Can you work these out from the drawing? Everything is in mm from the part's minimum corner. Give positions to 0.01 mm unless a question says otherwise; leave off trailing zeros. Write each loop counter-clockwise with the first axis right and the second up, starting at its lowest first coordinate (ties: lowest second). Pieces come first, ordered by that corner, then holes. Notation, with made-up numbers: (9.5, 51) -> (15.5, 51) arc R26 cw to (15.5, 79) -> close; hole circle Ø5 at (15.5, 79). An arc over 180 degrees is marked (long way). Return JSON: item names as keys, results as strings.
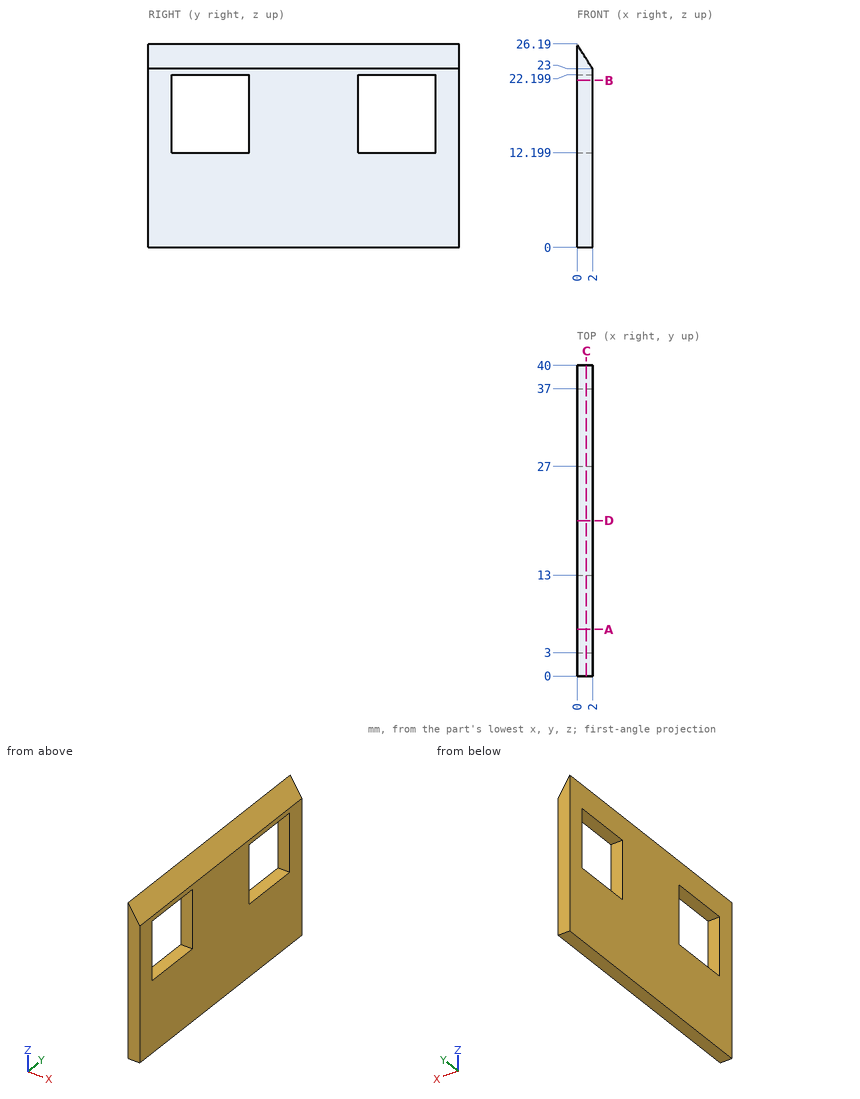
1. If I drill on line 1 (Y direction, x = 1.85, z = 16); line 2 (Z direction, x = 0.25, y = 33); line 3 (Z direction, x = 1, y = 11.5) (1 decimal), over which ranges is the centre line in solid material (lowest first)? Write a range as [from, to].
Taken from the geometry:
{"line 1": "y = [0, 3], [13, 27], [37, 40]", "line 2": "z = [0, 12.2], [22.2, 25.79]", "line 3": "z = [0, 12.2], [22.2, 24.6]"}
2. For pin 1 Ø0.6 at (x, y) = (1, 34.5) entering from +Z (1 decimal), with a flat end and sliding along its axis, tell me the tip position at first contact or that it passes through.
Taken from the geometry:
{"pin 1": "stops at z = 25.1"}
3. Suppose I cut it at D-D, the plane y = 20. List the corners of the cut face in (x, z) for me.
Taken from the geometry:
{"outline": "(0, 0) -> (2, 0) -> (2, 23) -> (0, 26.19) -> close"}
4. Suppose I cut it at B-B, the plane z = 21.5. List the corners of the cut face in (x, y) for me, and give its area (3 significant figures).
Taken from the geometry:
{"outline": "(0, 0) -> (2, 0) -> (2, 3) -> (0, 3) -> close; (0, 13) -> (2, 13) -> (2, 27) -> (0, 27) -> close; (0, 37) -> (2, 37) -> (2, 40) -> (0, 40) -> close", "area": "40.0 mm²"}
5. Suppose I cut it at A-A, the plane y = 6. List the corners of the cut face in (x, z) for me.
Taken from the geometry:
{"outline": "(0, 0) -> (2, 0) -> (2, 12.2) -> (0, 12.2) -> close; (0, 22.2) -> (2, 22.2) -> (2, 23) -> (0, 26.19) -> close"}
6. Suppose I cut it at C-C, the plane x = 1.2. List the corners of the cut face in (y, z) for me (1 decimal).
Taken from the geometry:
{"outline": "(0, 0) -> (40, 0) -> (40, 24.3) -> (0, 24.3) -> close; hole (3, 12.2) -> (13, 12.2) -> (13, 22.2) -> (3, 22.2) -> close; hole (27, 12.2) -> (37, 12.2) -> (37, 22.2) -> (27, 22.2) -> close"}
